from build123d import *

# Parameters (mm, degrees)
SKETCH1_W               = 50
SKETCH1_H               = 40
BOSS_EXTRUDE1_DEPTH     = 5
CUT_EXTRUDE1_DEPTH      = 21
CUT_EXTRUDE1_DEPTH_BACK = 21
CUT_EXTRUDE2_DEPTH      = 26
CUT_EXTRUDE2_DEPTH_BACK = 26
SKETCH4_W               = 3
SKETCH4_H               = 3
CUT_EXTRUDE3_DEPTH      = 26
CUT_EXTRUDE3_DEPTH_BACK = 26


with BuildPart() as part:
    # Sketch1 → Boss-Extrude1 (new body)
    with BuildSketch(Plane.XY):
        Rectangle(SKETCH1_W, SKETCH1_H)
    extrude(amount=BOSS_EXTRUDE1_DEPTH)

    # Sketch2 → Cut-Extrude1 (cut, two sides)
    with BuildSketch(Plane(origin=(0, 0, 0), x_dir=(1, 0, 0), z_dir=(0, 1, 0))) as cut_extrude1_sk:
        Polygon((-25, 0), (-20, -5), (-25, -5), align=None)
        Polygon((25, 0), (20, -5), (25, -5), align=None)
    extrude(amount=CUT_EXTRUDE1_DEPTH, mode=Mode.SUBTRACT)
    extrude(cut_extrude1_sk.sketch, amount=-CUT_EXTRUDE1_DEPTH_BACK, mode=Mode.SUBTRACT)

    # Sketch3 → Cut-Extrude2 (cut, two sides)
    with BuildSketch(Plane(origin=(0, 0, 0), x_dir=(0, 0, -1), z_dir=(1, 0, 0))) as cut_extrude2_sk:
        Polygon((0, -20), (-5, -15.916820135), (-5, -20), align=None)
    extrude(amount=CUT_EXTRUDE2_DEPTH, mode=Mode.SUBTRACT)
    extrude(cut_extrude2_sk.sketch, amount=-CUT_EXTRUDE2_DEPTH_BACK, mode=Mode.SUBTRACT)

    # Sketch4 → Cut-Extrude3 (cut, two sides)
    with BuildSketch(Plane(origin=(0, 0, 0), x_dir=(0, 0, -1), z_dir=(1, 0, 0))) as cut_extrude3_sk:
        with Locations((-3.5, 15)):
            Rectangle(SKETCH4_W, SKETCH4_H)
    extrude(amount=CUT_EXTRUDE3_DEPTH, mode=Mode.SUBTRACT)
    extrude(cut_extrude3_sk.sketch, amount=-CUT_EXTRUDE3_DEPTH_BACK, mode=Mode.SUBTRACT)


solid = part.part
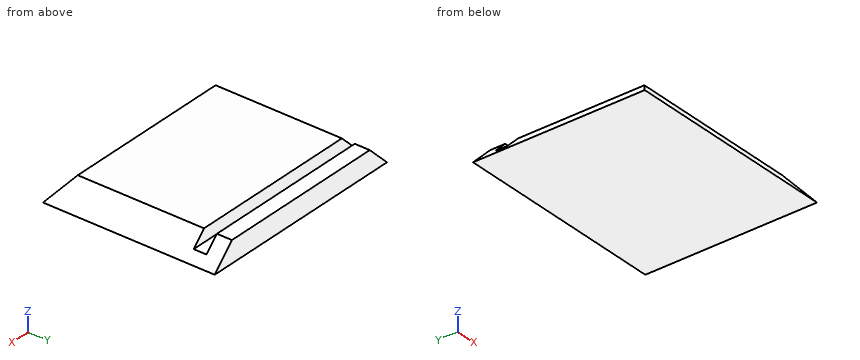
Here's how the part is built. I have some questions about the finished solid (model axes, mm). Coordinates: 2 decimals unless noted, no trailing zeros. Write each loop counter-clockwise with the first axis right and the second up, starting at its lowest first coordinate (ties: lowest second). Pieces come first, ordered by that corner, then holes.
Item 1: I want a section at A-A on z = 4.4. Write out the boundary of the cut face in (x, y).
Item 2: I want a section at C-C on y = 15. Write out the boundary of the cut face in (x, z).
Item 3: Will these pins go through, and if not, where does the flat tip stop? pin 1 (1 mm diameter, centred on y = 4, z = 1.5, fed in from +X); pin 2 (1 mm diameter, centred on x = -15, z = 1.5, fed in from -Y); pin 3 (2 mm diameter, centred on x = -9, z = 3, fed in from -Y).
Item 4: I want a section at D-D on z = 1. Write out the boundary of the cut face in (x, y).
Item 5: I want a section at B-B on x = -9. Write out the boundary of the cut face in (y, z), and give its area (3 significant figures).
Item 6: If I drill on line 1 (Y direction, x = 6.5, z = 4.75); line 2 (Y direction, x = -1, z = 2.4); line 3 (Z direction, x = -7, y = 15), over which ranges is the centre line in solid material (lowest first)?
Findings below:
1. outline: (-20.6, -16.41) - (20.6, -16.41) - (20.6, 13.5) - (-20.6, 13.5) - close; (-20.6, 16.5) - (20.6, 16.5) - (20.6, 20) - (-20.6, 20) - close
2. outline: (-25, 0) - (25, 0) - (23, 2) - (-23, 2) - close
3. pin 1: stops at x = 24
3. pin 2: stops at y = -19.18
3. pin 3: stops at y = -18.37
4. outline: (-24, -19.18) - (24, -19.18) - (24, 20) - (-24, 20) - close
5. outline: (-20, 0) - (20, 0) - (20, 5) - (16.5, 5) - (16.5, 2) - (13.5, 2) - (13.5, 5) - (-15.92, 5) - close
5. area: 181 mm2
6. line 1: y = -16.12 to 13.5, 16.5 to 20
6. line 2: y = -18.04 to 13.5, 16.5 to 20
6. line 3: z = 0 to 2
